```python
from build123d import *

# Parameters (mm, degrees)
F0_W      = 24
F0_H      = 15
F1_DEPTH  = 16
F2_T      = -2
F4_DEPTH  = 5
F5_W      = 5
F5_H      = 2
F6_DEPTH  = 20
F7_R      = 0.99999
F8_W      = 8.5
F8_H      = 2
F9_DEPTH  = 8
F10_DEPTH = 5
F12_DEPTH = 25
F13_R     = 2
F15_DEPTH = 2


# Not quite as in the source:
# - a fillet or chamfer is up to 0.001 mm smaller than in the source, because OpenCascade refuses the exact size


with BuildPart() as f1:
    # F0 (on Top) → F1 (new body)
    with BuildSketch(Plane.XY):
        Rectangle(F0_W, F0_H)
    extrude(amount=F1_DEPTH)

    # F2
    f2_openings = [f1.faces().sort_by_distance(p)[0] for p in [
        (0, 0, 16),
    ]]
    offset(amount=F2_T, openings=f2_openings)

    # F3 (on face) → F4 (cut)
    with BuildSketch(Plane.XZ.offset(7.5)):
        with BuildLine():
            Line((-2, 16), (-2, 13.25))
            ThreePointArc((-2, 13.25), (0, 5.25), (2, 13.25))
            Line((2, 13.25), (2, 16))
            Line((2, 16), (-2, 16))
        make_face()
    extrude(amount=-F4_DEPTH, mode=Mode.SUBTRACT)

    # F5 (on face) → F6 (join)
    with BuildSketch(Plane.XY.offset(16)):
        with Locations((-2, 6.5)):
            Rectangle(F5_W, F5_H)
    extrude(amount=F6_DEPTH)

    # F7 (radius 1 in the source; OpenCascade refuses exactly that, so slightly less here)
    f7_edges = [f1.edges().sort_by_distance(p)[0] for p in [
        (0.5, 5.5, 26),
        (0.5, 7.5, 26),
        (-4.5, 5.5, 26),
        (-4.5, 7.5, 26),
    ]]
    fillet(f7_edges, radius=F7_R)

    # F8 (on face) → F9 (cut)
    with BuildSketch(Plane.XY.offset(16)):
        with Locations((5.75, 6.5)):
            Rectangle(F8_W, F8_H)
    extrude(amount=-F9_DEPTH, mode=Mode.SUBTRACT)

    # F10 (add): a face of the model
    f10_faces = [f1.faces().sort_by_distance(p)[0] for p in [
        (0, 0, 0),
    ]]
    extrude(f10_faces, amount=F10_DEPTH)

    # F11 (on face) → F12 (cut)
    with BuildSketch(Plane.YZ.offset(12)):
        Polygon((7.5, -0.9807621135), (-7.5, -5), (7.5, -5), align=None)
    extrude(amount=-F12_DEPTH, mode=Mode.SUBTRACT)

    # F13
    f13_edges = [f1.edges().sort_by_distance(p)[0] for p in [
        (12, -7.5, 5.5),
        (-12, -7.5, 5.5),
        (-12, 7.5, 7.509619),
        (12, 7.5, 7.509619),
    ]]
    fillet(f13_edges, radius=F13_R)

    # F14 (on face) → F15 (cut)
    with BuildSketch(Plane(origin=(0, 7.5, 0), x_dir=(-1, 0, 0), z_dir=(0, 1, 0))):
        with BuildLine():
            add(Edge.make_bspline(
                [(-10, 4.0192378865), (-10, 2.0192378865), (-6.5, 2.0192378865), (-3, 2.0192378865), (-3, 4.0192378865)],
                knots=[3.1415926536, 3.1415926536, 3.1415926536, 4.7123889804, 4.7123889804, 6.2831853072, 6.2831853072, 6.2831853072], degree=2, weights=[1, 0.7071067812, 1, 0.7071067812, 1]))
            add(Edge.make_bspline(
                [(-3, 4.0192378865), (-3, 6.0192378865), (-6.5, 6.0192378865), (-10, 6.0192378865), (-10, 4.0192378865)],
                knots=[0, 0, 0, 1.5707963268, 1.5707963268, 3.1415926536, 3.1415926536, 3.1415926536], degree=2, weights=[1, 0.7071067812, 1, 0.7071067812, 1]))
        make_face()
    extrude(amount=-F15_DEPTH, mode=Mode.SUBTRACT)


solid = f1.part
```
Can you work these out from the model? Positions are in its coordinate system, mm. A direction names the side the tool comes from. Coordinates: 2 decimals unless noted, no trailing zeros. Order: outer loops, then holes, each group sorted by start corner. A loop starts at its lowest first (then second) coordinate and runs counter-clockwise, first axis right, second up. Notation, with made-up numbers: (-23.75, -12) - (14.25, -12) arc R31 ccw to (14.25, 13) - close; hole circle Ø5 at (80.5, 53.25). An arc over 180 degrees is marked (long way). Answer in a Markdown table with one row per item.
1. Suppose I cut it at C-C (x = -8.5). Please give me the cut outline in (y, z).
Reply:
| item | result |
|---|---|
| outline | (-7.5, -5) - (7.5, -0.98) - (7.5, 16) - (5.5, 16) - (5.5, 2) - (-5.5, 2) - (-5.5, 16) - (-7.5, 16) - close |
2. If we mould it in two halves opening along Y, with no side actions, what happens to faces 1 (the flat face through (-2, 5.5, 11)), 2 (the flat face through (-2, 7.5, 10)), 3 (the flat face through (6, 7, 8))? For each: pulls with the +Y half, pulls with the -Y half, needs draft (parallel to the pull), parting line crosses it, or undercut.
Reply:
| item | result |
|---|---|
| face 1 | undercut |
| face 2 | pulls with the +Y half |
| face 3 | needs draft |
3. Suppose I cut it at D-D (z = 9.5). Please give me the cut outline in (x, y), and give its area (3 significant figures).
Reply:
| item | result |
|---|---|
| outline | (-12, -5.5) arc R2 ccw to (-10, -7.5) - (-4.25, -7.5) - (-4.25, -5.5) - (-10, -5.5) - (-10, 5.5) - (1.5, 5.5) - (1.5, 7.5) - (-10, 7.5) arc R2 ccw to (-12, 5.5) - close; (4.25, -7.5) - (10, -7.5) arc R2 ccw to (12, -5.5) - (12, 5.5) arc R2 ccw to (10, 7.5) - (10, -5.5) - (4.25, -5.5) - close |
| area | 103 mm^2 |
4. If I drill on line 1 along X through (y, z) = (-2.5, 8.5); line 2 along Y through (x, z) = (-7.5, 3); line 3 along X through (y, z) = (-5.85, 9.5), over which ranges is the centre line in solid material (lowest first)?
Reply:
| item | result |
|---|---|
| line 1 | x = -12 to -10, 10 to 12 |
| line 2 | y = -7.5 to -5.5, 5.5 to 7.5 |
| line 3 | x = -11.97 to -4.25, 4.25 to 11.97 |
5. For pin 1 (9 mm diameter, centred on x = 2, y = 0.5, fed in from +Z); pin 2 (4 mm diameter, centred on x = -2, z = 27.5, fed in from -Y); pin 3 (1 mm diameter, centred on x = 5.5, y = 7, fed in from +Z), each with a flat end and sliding along its axis, tell me the tip position at first contact or that it passes through.
Reply:
| item | result |
|---|---|
| pin 1 | stops at z = 2 |
| pin 2 | stops at y = 5.5 |
| pin 3 | stops at z = 8 |
6. Suppose I cut it at B-B (x = -2.75). Please give me the cut outline in (y, z).
Reply:
| item | result |
|---|---|
| outline | (-7.5, -5) - (7.5, -0.98) - (7.5, 36) - (5.5, 36) - (5.5, 2) - (-5.5, 2) - (-5.5, 6.26) - (-7.5, 6.26) - close; (-7.5, 12.74) - (-5.5, 12.74) - (-5.5, 16) - (-7.5, 16) - close |
7. For faces 4 (the flat face through (-2, -7, 15)), 5 (the flat face through (-2.4, -5.5, 5.8)), 6 (the cylindrical face through (-0.158, -6.514, 5.253)), which set-ups out of +Z, -Z, +X, -X, +Y, -Y let a thin tool reach every point of the face, with its end or its side?
Reply:
| item | result |
|---|---|
| face 4 | +Z, -Y |
| face 5 | +Z |
| face 6 | -Y |
8. Suppose I cut it at A-A (z = 15.5). Please give me the cut outline in (x, y).
Reply:
| item | result |
|---|---|
| outline | (-12, -5.5) arc R2 ccw to (-10, -7.5) - (-2, -7.5) - (-2, -5.5) - (-10, -5.5) - (-10, 5.5) - (1.5, 5.5) - (1.5, 7.5) - (-10, 7.5) arc R2 ccw to (-12, 5.5) - close; (2, -7.5) - (10, -7.5) arc R2 ccw to (12, -5.5) - (12, 5.5) arc R2 ccw to (10, 7.5) - (10, -5.5) - (2, -5.5) - close |
